```python
from build123d import *

# Parameters (mm, degrees)
SKETCH1_R           = 1.5
BOSS_EXTRUDE1_DEPTH = 4
SKETCH2_W           = 8
SKETCH2_H           = 20
CUT_EXTRUDE1_DEPTH  = 1
FILLET1_R           = 1.5


with BuildPart() as part:
    # Sketch1 → Boss-Extrude1 (new body)
    with BuildSketch(Plane.XY):
        Polygon((23, 23), (23, 17), (78, 17), (78, 20), (84, 20), (84, 0), (0, 0), (0, 20), (8, 20), (8, 23), align=None)
        with Locations((3, 16)):
            Circle(SKETCH1_R, mode=Mode.SUBTRACT)
        with Locations((81, 16)):
            Circle(SKETCH1_R, mode=Mode.SUBTRACT)
        with Locations((3, 4)):
            Circle(SKETCH1_R, mode=Mode.SUBTRACT)
        with Locations((81, 4)):
            Circle(SKETCH1_R, mode=Mode.SUBTRACT)
    extrude(amount=BOSS_EXTRUDE1_DEPTH)

    # Sketch2 → Cut-Extrude1 (cut)
    with BuildSketch(Plane.XY.offset(4)):
        with Locations((4, 10)):
            Rectangle(SKETCH2_W, SKETCH2_H)
        with Locations((80, 10)):
            Rectangle(SKETCH2_W, SKETCH2_H)
    extrude(amount=-CUT_EXTRUDE1_DEPTH, mode=Mode.SUBTRACT)

    # Fillet1
    fillet1_edges = [part.edges().sort_by_distance(p)[0] for p in [
        (78, 17, 1.5),
        (23, 17, 2),
        (23, 23, 2),
        (8, 23, 2),
        (8, 20, 1.5),
    ]]
    fillet(fillet1_edges, radius=FILLET1_R - 0.0001)  # a hair under: the kernel refuses the full size


solid = part.part
```
Read the model definition and answer for the solid it produces. Units are mm, in the model's axes. A direction names the side the tool comes from. Give positions to 0.01 mm unless a question says otherwise; leave off trailing zeros. Order: outer loops, then holes, each group sorted by start corner. A loop starts at its lowest first (then second) coordinate and runs counter-clockwise, first axis right, second up.
(1) For faces 1 (the flat face through (4, 9, 3)), 2 (the flat face through (3, 20, 1)), 3 (the flat face through (78, 19, 1)), determine the directions among +Z, -Z, +X, -X, +Y, -Y from which every point of the face is accessible in a straight line to the end or side of a thin tool.
(2) Find section A-A (x = 81). Give the vertices of the cut face in (y, z), plus the area to 3 significant figures.
(3) Find section B-B (y = 4). Give the vertices of the cut face in (x, z).
(4) For a pull along Z with two mould halves and no side action, classify faces 4 (the flat face through (43, 9, 0)), 5 (the cylindrical face through (23.43, 17.45, 2.03)), 6 (the flat face through (42, 9, 4)) as released by +Z, released by -Z, zero draft, split by the parting line, or undercut.
(5) Find section D-D (y = 12.5). Give the vertices of the cut face in (x, z), plus the area to 3 significant figures.
(6) Straight lines are drawn through the part: L1, parallel to Y at x = 3, z = 2.45; L2, parallel to X at y = 4, z = 2.35; L3, parallel to Y at x = 65.5, z = 3.25. For each, find the intervals that lie inside material, in ascending order.
(7) Find section C-C (z = 1.15). Give the number of separate pieces and of enclosed holes in the cut face, plus the area to 3 significant figures.
(8) Given pin 1 (1.5 mm diameter, centred on x = 80, z = 2, fed in from +Y); pin 2 (1.2 mm diameter, centred on x = 59.5, z = 2, fed in from +Y); pin 3 (0.5 mm diameter, centred on y = 11.5, z = 3.5, fed in from +X); pin 4 (1.8 mm diameter, centred on x = 3, y = 16, fed in from +Z), each flat-ended and moving along its own axis, determine where each tip first touches the part or whether it passes through.
Result sheet:
1. face 1: +Z, -X, +Y, -Y
1. face 2: +Z, -Z, -X, +Y
1. face 3: +Z, -Z, +Y
2. outline: (0, 0) - (2.5, 0) - (2.5, 3) - (0, 3) - close; (5.5, 0) - (14.5, 0) - (14.5, 3) - (5.5, 3) - close; (17.5, 0) - (20, 0) - (20, 3) - (17.5, 3) - close
2. area: 42.0 mm2
3. outline: (0, 0) - (1.5, 0) - (1.5, 3) - (0, 3) - close; (4.5, 0) - (79.5, 0) - (79.5, 3) - (76, 3) - (76, 4) - (8, 4) - (8, 3) - (4.5, 3) - close; (82.5, 0) - (84, 0) - (84, 3) - (82.5, 3) - close
4. face 4: released by -Z
4. face 5: zero draft
4. face 6: released by +Z
5. outline: (0, 0) - (84, 0) - (84, 3) - (76, 3) - (76, 4) - (8, 4) - (8, 3) - (0, 3) - close
5. area: 320 mm2
6. L1: y = 0 to 2.5, 5.5 to 14.5, 17.5 to 20
6. L2: x = 0 to 1.5, 4.5 to 79.5, 82.5 to 84
6. L3: y = 0 to 17
7. separate pieces: 1
7. enclosed holes: 4
7. area: 1,530 mm2
8. pin 1: stops at y = 20
8. pin 2: stops at y = 17
8. pin 3: stops at x = 76
8. pin 4: passes through
